Check sheet for the modelled part. Datum: model origin and axes. Units: mm. Face numbers are marked on the shaded views. Round coordinates to 2 decimals unless told otherwise and drop trailing zeros. Loops run counter-clockwise (first coordinate to the right, second up) from the corner with the lowest first, then second, coordinate; pieces in that order, holes last. Notation, with made-up numbers: (27.5, -31) -> (55.5, -31) arc R17 cw to (55.5, -17) -> close; hole circle Ø5 at (-9, 49). An arc over 180 degrees is marked (long way). Use one line per item in the form item = value. Start each with the question number.
(1) Go/stop test with flat-tipped pins: pin 1 (12 mm diameter, centred on x = -17, y = 0.5, fed in from +Z); pin 2 (4 mm diameter, centred on y = -7, z = 5, fed in from +X); pin 3 (1 mm diameter, centred on x = 8.5, z = 2.5, fed in from +Y); pin 4 (6.5 mm diameter, centred on x = -18.25, y = 0, fed in from +Z). Record where each tip stops, or that it passes through.
(2) Draft check along X on the marked faces 1, 2 and 3. Enter one of: released by +X, released by -X, zero draft, split by the parting line, or undercut.
(3) Sectioned sample at B-B (y = 0). Record the cut outline in (x, z), and give its area (3 significant figures).
(4) Sectioned sample at A-A (x = 0). Record the cut outline in (y, z), and give its area (3 significant figures).
(5) Sectioned sample at D-D (y = 11.5). Record the cut outline in (x, z).
(6) Material ranges on probe 1 along Y at (x, z) = (0, 5.25); probe 2 along X at (y, z) = (-1.5, 1); probe 3 along Z at (x, y) = (13.5, -5), recorded low to high. Write a range as [from, to].
(7) Sectioned sample at C-C (z = 1.25). Record the cut outline in (x, y), and give its area (3 significant figures).
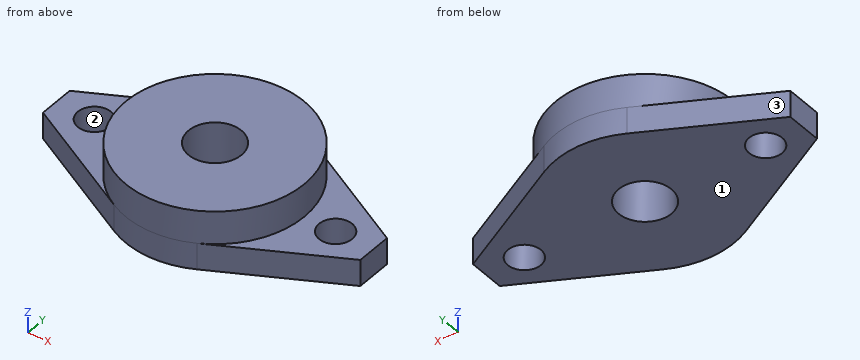
from build123d import *

# Parameters (mm, degrees)
CROQUIS1_R              = 2.5
CROQUIS1_R_2            = 4
SALIENTE_EXTRUIR1_DEPTH = 4
CROQUIS2_R              = 13.5
CROQUIS2_R_2            = 4
SALIENTE_EXTRUIR2_DEPTH = 5


with BuildPart() as part:
    # Croquis1 → Saliente-Extruir1 (new body)
    with BuildSketch(Plane.XY):
        with BuildLine():
            Line((24, 2.678571429), (24, -2.678571429))
            Line((24, -2.678571429), (6.258759048, -11.961518933))
            ThreePointArc((6.258759048, -11.961518933), (0, -13.5), (-6.258759048, -11.961518933))
            Line((-6.258759048, -11.961518933), (-24, -2.678571429))
            Line((-24, -2.678571429), (-24, 2.678571429))
            Line((-24, 2.678571429), (-6.258759048, 11.961518933))
            ThreePointArc((-6.258759048, 11.961518933), (0, 13.5), (6.258759048, 11.961518933))
            Line((6.258759048, 11.961518933), (24, 2.678571429))
        make_face()
        with Locations((18.25, 0)):
            Circle(CROQUIS1_R, mode=Mode.SUBTRACT)
        with Locations(Location((-18.25, 0, 0), (0, 0, 180))):
            Circle(CROQUIS1_R, mode=Mode.SUBTRACT)
        Circle(CROQUIS1_R_2, mode=Mode.SUBTRACT)
    extrude(amount=SALIENTE_EXTRUIR1_DEPTH)

    # Croquis2 → Saliente-Extruir2 (add)
    with BuildSketch(Plane.XY.offset(4)):
        with Locations(Location((0, 0, 0), (0, 0, 117.620415862))):
            Circle(CROQUIS2_R)
        Circle(CROQUIS2_R_2, mode=Mode.SUBTRACT)
    extrude(amount=SALIENTE_EXTRUIR2_DEPTH)


solid = part.part
Checks:
q1.pin_1 = 9
q1.pin_2 = 19.05
q1.pin_3 = 11.05
q1.pin_4 = 4
q2.face_1 = zero draft
q2.face_2 = undercut
q2.face_3 = released by -X
q3.outline = (-24, 0) -> (-20.75, 0) -> (-20.75, 4) -> (-24, 4) -> close; (-15.75, 0) -> (-4, 0) -> (-4, 9) -> (-13.5, 9) -> (-13.5, 4) -> (-15.75, 4) -> close; (4, 0) -> (15.75, 0) -> (15.75, 4) -> (13.5, 4) -> (13.5, 9) -> (4, 9) -> close; (20.75, 0) -> (24, 0) -> (24, 4) -> (20.75, 4) -> close
q3.area = 215 mm2
q4.outline = (-13.5, 0) -> (-4, 0) -> (-4, 9) -> (-13.5, 9) -> close; (4, 0) -> (13.5, 0) -> (13.5, 9) -> (4, 9) -> close
q4.area = 171 mm2
q5.outline = (-7.14, 0) -> (7.14, 0) -> (7.14, 4) -> (7.07, 4) -> (7.07, 9) -> (-7.07, 9) -> (-7.07, 4) -> (-7.14, 4) -> close
q6.probe_1 = [-13.5, -4], [4, 13.5]
q6.probe_2 = [-24, -20.25], [-16.25, -3.71], [3.71, 16.25], [20.25, 24]
q6.probe_3 = [0, 4]
q7.outline = (-24, -2.68) -> (-6.26, -11.96) arc R13.5 ccw to (6.26, -11.96) -> (24, -2.68) -> (24, 2.68) -> (6.26, 11.96) arc R13.5 ccw to (-6.26, 11.96) -> (-24, 2.68) -> close; hole circle Ø5 at (-18.25, 0); hole circle Ø8 at (0, 0); hole circle Ø5 at (18.25, 0)
q7.area = 755 mm2
